from build123d import *

# Parameters (mm, degrees)
SKETCH1_R               = 2.159
BOSS_EXTRUDE1_DEPTH     = 2.54
FILLET2_R               = 2.54
FILLET3_R               = 0.0254
CUT_EXTRUDE1_DEPTH      = 8.536089729
CUT_EXTRUDE1_DEPTH_BACK = 8.536089729
SKETCH6_R               = 0.635


with BuildPart() as part:
    # Sketch1 → Boss-Extrude1 (new body)
    with BuildSketch(Plane.XY):
        with BuildLine():
            Line((1.03203613, 3.002586623), (4.689867375, 0.484445873))
            ThreePointArc((4.689867375, 0.484445873), (5.512880678, 0.206373406), (6.374728135, 0.097313081))
            ThreePointArc((6.374728135, 0.097313081), (3.49593357, -2.139961579), (0, -3.175))
            ThreePointArc((0, -3.175), (-3.131600033, 0.523169415), (1.03203613, 3.002586623))
        make_face()
        Circle(SKETCH1_R, mode=Mode.SUBTRACT)
    extrude(amount=BOSS_EXTRUDE1_DEPTH)

    # Fillet2
    fillet2_edges = [part.edges().sort_by_distance(p)[0] for p in [
        (1.03203613, 3.002586623, 1.27),
        (0, -3.175, 1.27),
    ]]
    fillet(fillet2_edges, radius=FILLET2_R)

    # Fillet3
    fillet3_edges = [part.edges().sort_by_distance(p)[0] for p in [
        (6.374728135, 0.097313081, 1.27),
    ]]
    fillet(fillet3_edges, radius=FILLET3_R)

    # Sketch6 → Cut-Extrude1 (cut, two sides: drawn at the far end of the back side and taken through both)
    with BuildSketch(Plane(origin=(0, 0, 0), x_dir=(1, 0, 0), z_dir=(0, 1, 0)).offset(-CUT_EXTRUDE1_DEPTH_BACK)):
        with Locations(Location((3.419867375, -1.27, 0), (0, 0, 270))):
            Circle(SKETCH6_R)
    extrude(amount=CUT_EXTRUDE1_DEPTH + CUT_EXTRUDE1_DEPTH_BACK, mode=Mode.SUBTRACT)


solid = part.part
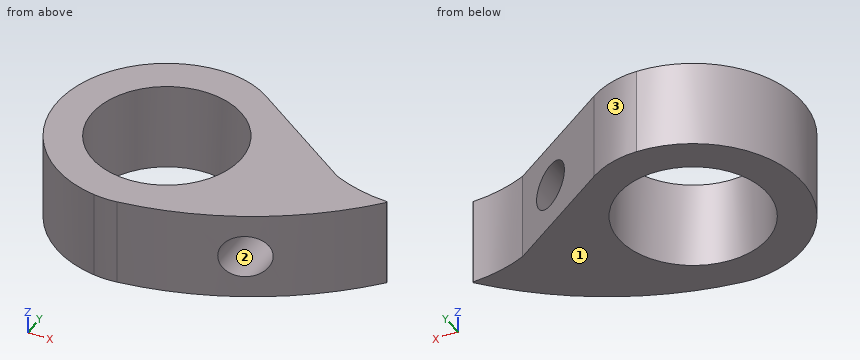
Design review of the part built by this model. Coordinates are the model's own, in mm. Face numbers are marked on the shaded views. Round coordinates to 2 decimals unless told otherwise and drop trailing zeros. Write each loop counter-clockwise with the first axis right and the second up, starting at its lowest first coordinate (ties: lowest second). Pieces come first, ordered by that corner, then holes. Notation, with made-up numbers: (-4, 46.25) -> (5, 46.25) arc R18 ccw to (5, 60.25) -> close; hole circle Ø7 at (8, 40.25). An arc over 180 degrees is marked (long way). One line per item, written item: value. Start each with the question number.
Q1. Insertion check: P1, Ø1.5, axis at x = 3.42, z = 1.27, coming from the +Y side (3 decimals); P2, Ø1, axis at x = -1.5, z = 1, coming from the -Y side. Each pin has a flat end and moves straight along its axis. Give the tip position at first contact, or say it passes through.
Q2. Add section A-A (y = -1.5). Give the boundary of the cut face in (x, z) (3 decimals), then the cut area to 3 significant figures.
Q3. Add section D-D (z = 1.3). State how many separate pieces and enclosed holes the cut face has, then the cut area to 3 significant figures.
Q4. To check wall thickness, follow probe 1 along X at (y, z) = (-1.1, 1.27); probe 2 along Y at (x, z) = (0, 1.85); probe 3 along X at (y, z) = (-1.5, 1.8). State the ranges of each line that lie inside material, in increasing order.
Q5. Add section B-B (y = 1.25). Give the boundary of the cut face in (x, z) (3 decimals).
Q6. The part is to be moulded in two halves that separate along Z. For the marked faces 1, 2 and 3, say which applies: pulls with the +Z half, pulls with the -Z half, needs draft (parallel to the pull), parting line crosses it, or undercut.
Q7. Add section C-C (x = 1.75). Give the boundary of the cut face in (y, z).
Response:
1. P1: stops at y = 1.875
1. P2: stops at y = -3.01
2. outline: (-2.798, 0) -> (-1.553, 0) -> (-1.553, 2.54) -> (-2.798, 2.54) -> close; (1.553, 0) -> (4.569, 0) -> (4.569, 2.54) -> (1.553, 2.54) -> close; hole circle Ø1.27 at (3.42, 1.27)
2. area: 9.56 mm^2
3. separate pieces: 2
3. enclosed holes: 1
3. area: 19.7 mm^2
4. probe 1: x = -2.98 to -1.86, 1.86 to 2.78, 4.05 to 5.11
4. probe 2: y = -3.17 to -2.16, 2.16 to 3.17
4. probe 3: x = -2.8 to -1.55, 1.55 to 3.07, 3.77 to 4.57
5. outline: (-2.919, 0) -> (-1.76, 0) -> (-1.76, 2.54) -> (-2.919, 2.54) -> close; (1.76, 0) -> (3.578, 0) -> (3.578, 0.655) arc R0.635 cw (long way) to (3.578, 1.885) -> (3.578, 2.54) -> (1.76, 2.54) -> close
6. face 1: pulls with the -Z half
6. face 2: undercut
6. face 3: needs draft
7. outline: (-2.83, 0) -> (-1.26, 0) -> (-1.26, 2.54) -> (-2.83, 2.54) -> close; (1.26, 0) -> (2.51, 0) -> (2.51, 2.54) -> (1.26, 2.54) -> close
